Geometry: final body of the model. Coordinates: model frame, mm. A direction names the side the tool comes from. Give positions to 0.01 mm unless a question says otherwise; leave off trailing zeros. Write each loop counter-clockwise with the first axis right and the second up, starting at its lowest first coordinate (ties: lowest second). Pieces come first, ordered by that corner, then holes. Notation, with made-up numbers: (31.5, 23) - (35.5, 23) arc R19 ccw to (35.5, 36) - close; hole circle Ø6 at (17, 8). An arc over 180 degrees is marked (long way). One line per question, with ' | ' between items. Start each with the question number.
```python
from build123d import *

# Parameters (mm, degrees)
BOSS_EXTRUDE2_DEPTH = 50.8
CUT_EXTRUDE2_DEPTH  = 63.5
CUT_EXTRUDE3_DEPTH  = 63.5
SKETCH3_R           = 5
BOSS_EXTRUDE3_DEPTH = 20


with BuildPart() as part:
    # Sketch1 → Boss-Extrude2 (new body)
    with BuildSketch(Plane.XY):
        Polygon((0, 0), (0, 76.2), (50.8, 76.2), (50.8, 0), (38.1, 0), (38.1, 50.8), (12.7, 50.8), (12.7, 0), align=None)
    extrude(amount=-BOSS_EXTRUDE2_DEPTH)

    # Sketch4 → Cut-Extrude2 (cut)
    with BuildSketch(Plane.XY):
        Polygon((0, 50.8), (12.7, 0), (0, 0), align=None)
    extrude(amount=-CUT_EXTRUDE2_DEPTH, mode=Mode.SUBTRACT)

    # Sketch5 → Cut-Extrude3 (cut)
    with BuildSketch(Plane.XY):
        Polygon((50.8, 50.8), (38.1, 0), (50.8, 0), align=None)
    extrude(amount=-CUT_EXTRUDE3_DEPTH, mode=Mode.SUBTRACT)

    # Sketch3 → Boss-Extrude3 (add)
    with BuildSketch(Plane(origin=(0, 76.2, 0), x_dir=(1, 0, 0), z_dir=(0, 1, 0))):
        with Locations((25.4, 25.8)):
            Circle(SKETCH3_R)
    extrude(amount=BOSS_EXTRUDE3_DEPTH)


solid = part.part
```
1) Section C-C, the plane x = 25.4. Output: boundary loops of the cut face in (y, z), plus the area to 3 significant figures.
2) Line query: L1, parallel to Y at x = 23, z = -45; L2, parallel to X at y = 39.5, z = -9.5 (3 decimals); L3, parallel to X at y = 25, z = -15.5. Output: solid intervals per line, ascending.
3) Section D-D, the plane z = -25.8. Output: boundary loops of the cut face in (x, y).
4) Section B-B, the plane z = -33. Output: boundary loops of the cut face in (x, y), plus the area to 3 significant figures.
5) First-contact query: pin 1 Ø2 at (y, z) = (65, -20.5) entering from -X; pin 2 Ø1 at (x, z) = (25.5, -27) entering from -Y; pin 3 Ø4 at (x, z) = (45.5, -26) entering from +Y; pin 4 Ø3 at (y, z) = (15.5, -13) entering from -X. Flat tips, straight axial feed; report the tip coordinate or a pass-through.
6) Pull-direction query (X, two-part tool) for faces 1 (the flat face through (0, 63, -25)), 2 (the flat face through (25, 96.2, -26)), 3 (the flat face through (38.1, 25, -25)); classes: +X half, -X half, draft (parallel to the pull), parting line (faces both ways), or undercut.
7) Reachability of faces 4 (the flat face through (26, 56, -50.8)), 5 (the cylindrical face through (24.749, 86.06, -30.757)), 6 (the flat face through (26, 50.8, -25)) from +Z, -Z, +X, -X, +Y, -Y: full face, straight path, thin tool, end or side. Return the list, or none.
8) Section A-A, the plane y = 25. Output: boundary loops of the cut face in (x, z).
Answer key:
1) outline: (50.8, -50.8) - (76.2, -50.8) - (76.2, -30.8) - (96.2, -30.8) - (96.2, -20.8) - (76.2, -20.8) - (76.2, 0) - (50.8, 0) - close | area: 1,490 mm^2
2) L1: 50.8 to 76.2 | L2: 2.825 to 12.7, 38.1 to 47.975 | L3: 6.45 to 12.7, 38.1 to 44.35
3) outline: (0, 50.8) - (12.7, 0) - (12.7, 50.8) - (38.1, 50.8) - (38.1, 0) - (50.8, 50.8) - (50.8, 76.2) - (30.4, 76.2) - (30.4, 96.2) - (20.4, 96.2) - (20.4, 76.2) - (0, 76.2) - close
4) outline: (0, 50.8) - (12.7, 0) - (12.7, 50.8) - (38.1, 50.8) - (38.1, 0) - (50.8, 50.8) - (50.8, 76.2) - (0, 76.2) - close | area: 1,940 mm^2
5) pin 1: x = 0 | pin 2: y = 50.8 | pin 3: y = 76.2 | pin 4: x = 8.45
6) face 1: -X half | face 2: draft | face 3: undercut
7) face 4: -Z, +X, -X, +Y, -Y | face 5: +Y | face 6: +Z, -Z, -Y
8) outline: (6.45, -50.8) - (12.7, -50.8) - (12.7, 0) - (6.45, 0) - close; (38.1, -50.8) - (44.35, -50.8) - (44.35, 0) - (38.1, 0) - close
